The model under review builds one solid part; all positions refer to its coordinate system, in mm. Face numbers are marked on the shaded views. A direction names the side the tool comes from. Round coordinates to 2 decimals unless told otherwise and drop trailing zeros. Order: outer loops, then holes, each group sorted by start corner. A loop starts at its lowest first (then second) coordinate and runs counter-clockwise, first axis right, second up. Notation, with made-up numbers: (57.5, -23.5) -> (81.5, -23.5) arc R22 cw to (81.5, -7.5) -> close; hole circle Ø11 at (-28.75, 50). An arc over 180 degrees is marked (long way). Use a Markdown table: item, result. Add a question column.
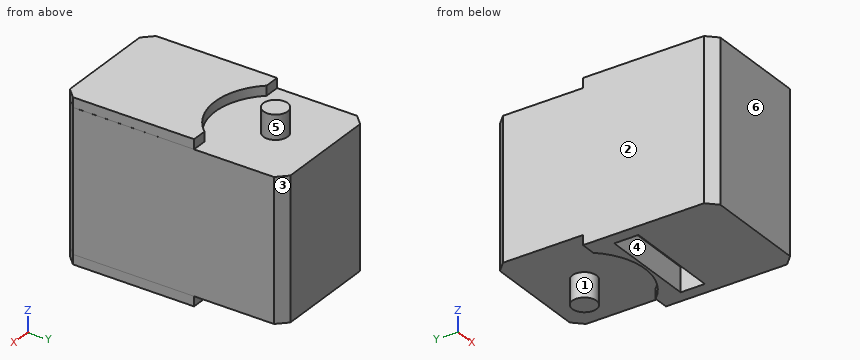
Autodesk Inventor part; units mm, degrees
ref_plane "YZ Plane" through (0, 0, 0) normal (1, 0, 0) x (0, 1, 0)
ref_plane "XZ Plane" through (0, 0, 0) normal (0, 1, 0) x (-1, 0, 0)
ref_plane "XY Plane" through (0, 0, 0) normal (0, 0, 1) x (1, 0, 0)
sketch "Sketch1" plane through (0, 0, 0) normal (0, 0, 1) x (1, 0, 0)
  line L0 (0, 0) -> (25, 0)
  line L1 (25, 0) -> (25, 45.5)
  line L2 (25, 45.5) -> (0, 45.5)
  line L3 (0, 45.5) -> (0, 0)
  dimension "d0" = 25
  dimension "d1" = 45.5
extrude "Extrusion1" add sketch "Sketch1" along normal blind 29
chamfer "Chamfer1" distance 2 angle 45 4 edges at (25, 45.5, 14.5) (0, 45.5, 14.5) (25, 0, 14.5) (0, 0, 14.5)
sketch "Sketch2" plane through (0, 0, 29) normal (0, 0, 1) x (1, 0, 0)
  line L0 (23, 45.5) -> (2, 45.5)
  line L1 (12.5, 45.5) -> (12.5, 0)
  line L2 (2, 0) -> (23, 0)
  line L3 (12.5, 22.75) -> (12.5, 35.25)
  circle A0 centre (12.5, 35.25) radius 12.5
  line L4 (12.5, 0) -> (2, 0)
  line L5 (0, 2) -> (2, 0)
  line L6 (2, 0) -> (0, 1.9914)
  line L7 (0, 1.9914) -> (0, 26.9914)
  line L8 (0, 43.5) -> (0, 2)
  line L9 (0, 26.9914) -> (3.1167, 26.9914)
  line L10 (12.5, 0) -> (23, 0)
  line L11 (23, 0) -> (24.9828, 1.9914)
  line L12 (24.9828, 1.9914) -> (23, 0)
  line L13 (24.9828, 1.9914) -> (25, 26.9914)
  line L14 (25, 2) -> (25, 43.5)
  line L15 (25, 26.9914) -> (21.8833, 26.9914)
  point P0 (0, 0)
  dimension "d8" = 12.5
  dimension "d9" = 25
  dimension "d10" = 25
extrude "Extrusion2" add sketch "Sketch2" along normal blind 2 contours L15 L13 L11 L2 L1 A0 | L1 L2 L5 L7 L9 A0
ref_plane "Work Plane1" through (0, 0, 14.5) normal (0, 0, 1) x (1, 0, 0)
sketch "Sketch3" plane through (0, 0, 29) normal (0, 0, 1) x (1, 0, 0)
  arc A0 (3.1167, 26.9914) -> (21.8833, 26.9914) centre (12.5, 35.25) ccw
  circle A1 centre (12.5, 35.25) radius 2.5
  point P0 (0, 0)
  dimension "d13" = 5
extrude "Extrusion3" add sketch "Sketch3" along normal blind 5
mirror "Mirror1" about plane through (0, 0, 14.5) normal (0, 0, 1) of "Extrusion2", "Extrusion3"
sketch "Sketch5" plane through (12.5, 35.25, -2) normal (0, 0, -1) x (-1, 0, 0)
  circle A0 centre (0, 0) radius 2.5
  line L0 (0, 0) -> (0, -13)
  line L1 (0, -13) -> (10, -13)
  line L2 (10, -13) -> (10, -18)
  line L3 (10, -18) -> (-10, -18)
  line L4 (-10, -18) -> (-10, -13)
  line L5 (-10, -13) -> (0, -13)
  point P0 (12.5, -35.25)
  dimension "d16" = 13
  dimension "d17" = 10
  dimension "d18" = 5
  dimension "d19" = 20
extrude "Extrusion4" cut sketch "Sketch5" against normal blind 5 contours L1 L2 L3 L4 L5
ref_plane "Work Plane2" through (0, 0, 14.5) normal (0, 0, 1) x (1, 0, 0)
properties part number "feetech_sc215"
Q1. For pin 1 (3 mm diameter, centred on x = 6, y = 37, fed in from +Z); pin 2 (1.5 mm diameter, centred on x = 9, y = 20.5, fed in from +Z); pin 3 (7.5 mm diameter, centred on x = 6.5, y = 13, fed in from -Z), all flat-tipped, find the tip position at first contact; note any pin that passes through.
Q2. Add section C-C, the plane x = 9.25. Give the boundary of the cut face in (y, z), then the cut area to 3 significant figures.
Q3. To check wall thickness, follow line 1 along Y through (x, z) = (14.75, -0.5); line 2 along Y through (x, z) = (16.25, 2); line 3 along Z through (x, y) = (4.5, 38.5). State the ranges of each line that lie inside material, in increasing order.
Q4. Add section A-A, the plane x = 12.5. Give the boundary of the cut face in (y, z), then the cut area to 3 significant figures.
Q5. Draft analysis for pull direction Y (two halves, no side actions). For the marked faces 1, 2, 3 and 4, state which applies: released by +Y, released by -Y, zero draft, split by the parting line, or undercut.
Q6. Add section B-B, the plane y = 35.25. Give the boundary of the cut face in (x, z), then the cut area to 3 significant figures.
Q7. For the marked faces 5 and 6, list the 3-axis set-ups (+Z, -Z, +X, -X, +Y, -Y) from which the entire face can be reached by the end or side of a thin tool; tool diameter is ignored.
Return value:
| question | item | result |
|---|---|---|
| 1 | pin 1 | z = 29 |
| 1 | pin 2 | z = 31 |
| 1 | pin 3 | z = -2 |
| 2 | outline | (0, -2) -> (17.25, -2) -> (17.25, 3) -> (22.25, 3) -> (22.25, -2) -> (23.18, -2) -> (23.18, 0) -> (45.5, 0) -> (45.5, 29) -> (23.18, 29) -> (23.18, 31) -> (0, 31) -> close |
| 2 | area | 1,390 mm² |
| 3 | line 1 | 0 to 17.25, 22.25 to 22.95, 34.16 to 36.34 |
| 3 | line 2 | 0 to 17.25, 22.25 to 45.5 |
| 3 | line 3 | 0 to 29 |
| 4 | outline | (0, -2) -> (17.25, -2) -> (17.25, 3) -> (22.25, 3) -> (22.25, -2) -> (22.75, -2) -> (22.75, 0) -> (32.75, 0) -> (32.75, -5) -> (37.75, -5) -> (37.75, 0) -> (45.5, 0) -> (45.5, 29) -> (37.75, 29) -> (37.75, 34) -> (32.75, 34) -> (32.75, 29) -> (22.75, 29) -> (22.75, 31) -> (0, 31) -> close |
| 4 | area | 1,440 mm² |
| 5 | face 1 | undercut |
| 5 | face 2 | zero draft |
| 5 | face 3 | released by +Y |
| 5 | face 4 | undercut |
| 6 | outline | (0, 0) -> (10, 0) -> (10, -5) -> (15, -5) -> (15, 0) -> (25, 0) -> (25, 29) -> (15, 29) -> (15, 34) -> (10, 34) -> (10, 29) -> (0, 29) -> close |
| 6 | area | 775 mm² |
| 7 | face 5 | +Z |
| 7 | face 6 | +Z, -Z, +X, -X, -Y |
